from build123d import *

# Parameters (mm, degrees)
SKETCH1_W           = 50
SKETCH1_H           = 32.926829268
BOSS_EXTRUDE1_DEPTH = 3
CUT_EXTRUDE1_REACH  = 61.943
SKETCH2_R           = 1
SKETCH2_R_2         = 5
CUT_EXTRUDE2_REACH  = 61.943
SKETCH3_R           = 2.5
FILLET1_R           = 1


with BuildPart() as part:
    # Sketch1 → Boss-Extrude1 (new body)
    with BuildSketch(Plane(origin=(0, 0, 0), x_dir=(1, 0, 0), z_dir=(0, 1, 0))):
        with Locations((25, 16.463414634)):
            Rectangle(SKETCH1_W, SKETCH1_H)
    extrude(amount=BOSS_EXTRUDE1_DEPTH)

    # Sketch2 → Cut-Extrude1 (cut, up to next)
    with BuildSketch(Plane(origin=(0, 3, 0), x_dir=(1, 0, 0), z_dir=(0, 1, 0)), mode=Mode.PRIVATE) as cut_extrude1_sk1:
        with Locations(Location((25, 8.963414634, 0), (0, 0, 270))):
            Circle(SKETCH2_R)
    cut_extrude1_tool1 = extrude(cut_extrude1_sk1.sketch, amount=-CUT_EXTRUDE1_REACH, mode=Mode.PRIVATE) & part.part
    # Sketch2 → Cut-Extrude1 (cut, up to next)
    with BuildSketch(Plane(origin=(0, 3, 0), x_dir=(1, 0, 0), z_dir=(0, 1, 0)), mode=Mode.PRIVATE) as cut_extrude1_sk2:
        with Locations(Location((25, 16.463414634, 0), (0, 0, 270))):
            Circle(SKETCH2_R_2)
    cut_extrude1_tool2 = extrude(cut_extrude1_sk2.sketch, amount=-CUT_EXTRUDE1_REACH, mode=Mode.PRIVATE) & part.part
    # Sketch2 → Cut-Extrude1 (cut, up to next)
    with BuildSketch(Plane(origin=(0, 3, 0), x_dir=(1, 0, 0), z_dir=(0, 1, 0)), mode=Mode.PRIVATE) as cut_extrude1_sk3:
        with Locations(Location((25, 23.963414634, 0), (0, 0, 270))):
            Circle(SKETCH2_R)
    cut_extrude1_tool3 = extrude(cut_extrude1_sk3.sketch, amount=-CUT_EXTRUDE1_REACH, mode=Mode.PRIVATE) & part.part
    add(cut_extrude1_tool1.solids().sort_by_distance((25, 3, -8.963415))[0], mode=Mode.SUBTRACT)
    add(cut_extrude1_tool2.solids().sort_by_distance((25, 3, -16.463415))[0], mode=Mode.SUBTRACT)
    add(cut_extrude1_tool3.solids().sort_by_distance((25, 3, -23.963415))[0], mode=Mode.SUBTRACT)

    # Sketch3 → Cut-Extrude2 (cut, up to next)
    with BuildSketch(Plane(origin=(0, 3, 0), x_dir=(1, 0, 0), z_dir=(0, 1, 0)), mode=Mode.PRIVATE) as cut_extrude2_sk1:
        with Locations(Location((43.5, 6.5, 0), (0, 0, 270))):
            Circle(SKETCH3_R)
    cut_extrude2_tool1 = extrude(cut_extrude2_sk1.sketch, amount=-CUT_EXTRUDE2_REACH, mode=Mode.PRIVATE) & part.part
    # Sketch3 → Cut-Extrude2 (cut, up to next)
    with BuildSketch(Plane(origin=(0, 3, 0), x_dir=(1, 0, 0), z_dir=(0, 1, 0)), mode=Mode.PRIVATE) as cut_extrude2_sk2:
        with Locations(Location((43.5, 26.426829268, 0), (0, 0, 270))):
            Circle(SKETCH3_R)
    cut_extrude2_tool2 = extrude(cut_extrude2_sk2.sketch, amount=-CUT_EXTRUDE2_REACH, mode=Mode.PRIVATE) & part.part
    # Sketch3 → Cut-Extrude2 (cut, up to next)
    with BuildSketch(Plane(origin=(0, 3, 0), x_dir=(1, 0, 0), z_dir=(0, 1, 0)), mode=Mode.PRIVATE) as cut_extrude2_sk3:
        with Locations(Location((6.5, 26.426829268, 0), (0, 0, 270))):
            Circle(SKETCH3_R)
    cut_extrude2_tool3 = extrude(cut_extrude2_sk3.sketch, amount=-CUT_EXTRUDE2_REACH, mode=Mode.PRIVATE) & part.part
    # Sketch3 → Cut-Extrude2 (cut, up to next)
    with BuildSketch(Plane(origin=(0, 3, 0), x_dir=(1, 0, 0), z_dir=(0, 1, 0)), mode=Mode.PRIVATE) as cut_extrude2_sk4:
        with Locations(Location((6.5, 6.5, 0), (0, 0, 270))):
            Circle(SKETCH3_R)
    cut_extrude2_tool4 = extrude(cut_extrude2_sk4.sketch, amount=-CUT_EXTRUDE2_REACH, mode=Mode.PRIVATE) & part.part
    add(cut_extrude2_tool1.solids().sort_by_distance((43.5, 3, -6.5))[0], mode=Mode.SUBTRACT)
    add(cut_extrude2_tool2.solids().sort_by_distance((43.5, 3, -26.426829))[0], mode=Mode.SUBTRACT)
    add(cut_extrude2_tool3.solids().sort_by_distance((6.5, 3, -26.426829))[0], mode=Mode.SUBTRACT)
    add(cut_extrude2_tool4.solids().sort_by_distance((6.5, 3, -6.5))[0], mode=Mode.SUBTRACT)

    # Fillet1
    fillet1_edges = [part.edges().sort_by_distance(p)[0] for p in [
        (50, 3, -16.463414634),
        (25, 3, -32.926829268),
        (0, 3, -16.463414634),
        (25, 0, -32.926829268),
        (50, 0, -16.463414634),
        (25, 0, 0),
        (0, 0, -16.463414634),
        (25, 3, 0),
        (0, 1.5, -32.926829268),
        (50, 1.5, -32.926829268),
        (50, 1.5, 0),
        (0, 1.5, 0),
    ]]
    fillet(fillet1_edges, radius=FILLET1_R)


solid = part.part
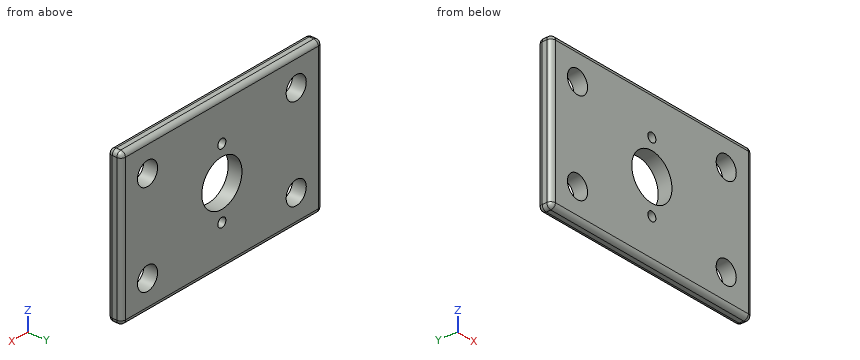
Model file for the job. Use its own axes, mm. Coordinates: 2 decimals unless noted, no trailing zeros. Order: outer loops, then holes, each group sorted by start corner. A loop starts at its lowest first (then second) coordinate and runs counter-clockwise, first axis right, second up. Notation, with made-up numbers: (36, 52.5) -> (43, 52.5) arc R24 ccw to (43, 81.5) -> close; hole circle Ø4 at (24.5, 31.25). An arc over 180 degrees is marked (long way). Return JSON: item names as keys, results as strings. Group by question number.
Item 1: Saw through at D-D on z = -20.5. Write the cut outline in (x, y).
Item 2: Saw through at B-B on x = 25. Write the cut outline in (y, z), then the cut area to 3 significant figures.
Item 3: Saw through at C-C on z = -6.5. Write the cut outline in (x, y), then the cut area to 3 significant figures.
Item 4: Saw through at A-A on x = 43.5. Write the cut outline in (y, z).
Item 5: Wall check: line 1 along X through (y, z) = (1.8, -6.5); line 2 along X through (y, z) = (1.7, -5.5); line 3 along Z through (x, y) = (23.5, 2.35). Give the ranges that are in metal, low to high. Write a range as [from, to].
Values found:
{
 "1": {"outline": "(0, 1) arc R1 ccw to (1, 0) -> (22.05, 0) -> (22.05, 3) -> (1, 3) arc R1 ccw to (0, 2) -> close; (27.95, 0) -> (49, 0) arc R1 ccw to (50, 1) -> (50, 2) arc R1 ccw to (49, 3) -> (27.95, 3) -> close"},
 "2": {"outline": "(0, -31.93) arc R1 ccw to (1, -32.93) -> (2, -32.93) arc R1 ccw to (3, -31.93) -> (3, -24.96) -> (0, -24.96) -> close; (0, -22.96) -> (3, -22.96) -> (3, -21.46) -> (0, -21.46) -> close; (0, -11.46) -> (3, -11.46) -> (3, -9.96) -> (0, -9.96) -> close; (0, -7.96) -> (3, -7.96) -> (3, -1) arc R1 ccw to (2, 0) -> (1, 0) arc R1 ccw to (0, -1) -> close", "area": "55.9 mm2"},
 "3": {"outline": "(0, 1) arc R1 ccw to (1, 0) -> (4, 0) -> (4, 3) -> (1, 3) arc R1 ccw to (0, 2) -> close; (9, 0) -> (41, 0) -> (41, 3) -> (9, 3) -> close; (46, 0) -> (49, 0) arc R1 ccw to (50, 1) -> (50, 2) arc R1 ccw to (49, 3) -> (46, 3) -> close", "area": "119 mm2"},
 "4": {"outline": "(0, -31.93) arc R1 ccw to (1, -32.93) -> (2, -32.93) arc R1 ccw to (3, -31.93) -> (3, -28.93) -> (0, -28.93) -> close; (0, -23.93) -> (3, -23.93) -> (3, -9) -> (0, -9) -> close; (0, -4) -> (3, -4) -> (3, -1) arc R1 ccw to (2, 0) -> (1, 0) arc R1 ccw to (0, -1) -> close"},
 "5": {"line 1": "x = [0, 4], [9, 41], [46, 50]", "line 2": "x = [0, 4.21], [8.79, 41.21], [45.79, 50]", "line 3": "z = [-32.86, -21.23], [-11.69, -0.06]"}
}
